Geometry: see drawing. Coordinates: mm, zero at the bounding-box minimum. A direction names the side the tool comes from. Give positions to 0.01 mm unless a question says otherwise; leave off trailing zeros. Write each loop counter-clockwise with the first axis right and the second up, starting at its lowest first coordinate (ties: lowest second). Pieces come first, ordered by that corner, then holes. Notation, with made-up numbers: (79, 89) -> (89, 89) arc R16 cw to (89, 99) -> close; hole circle Ø9 at (88.25, 84). An arc over 180 degrees is marked (long way). Use CSV: the item, a comma, the result in double quotes. Start each with the question number.
1) Section D-D (y = 21.5). Output: boundary loops of the cut face in (x, z), plus the area to 3 significant figures.
2) Set-up query: the marked faces 1, 2 and 3. Return all of +Z, -Z, +X, -X, +Y, -Y with unobstructed straight access to the full face (end or side cutting, diameter ignored); none if empty.
3) Section A-A (z = 21.5). Output: boundary loops of the cut face in (x, y).
4) Contact query for flat-ended pins moving along their axis: P1, Ø5, axis at x = 6, z = 19.5, coming from the +Y side; P2, Ø2, axis at x = 16, z = 18.5, coming from the -Y side; P3, Ø5, axis at x = 5, y = 29.5, coming from the +Z side. Output: stop coordinate, or through.
5) Section B-B (x = 31.5). Output: boundary loops of the cut face in (y, z), plus the area to 3 significant figures.
6) Material intervals for line 1 (Y direction, x = 8.5, z = 20); line 2 (Y direction, x = 47, z = 24.5), sorted ascending. Write a range as [from, to].
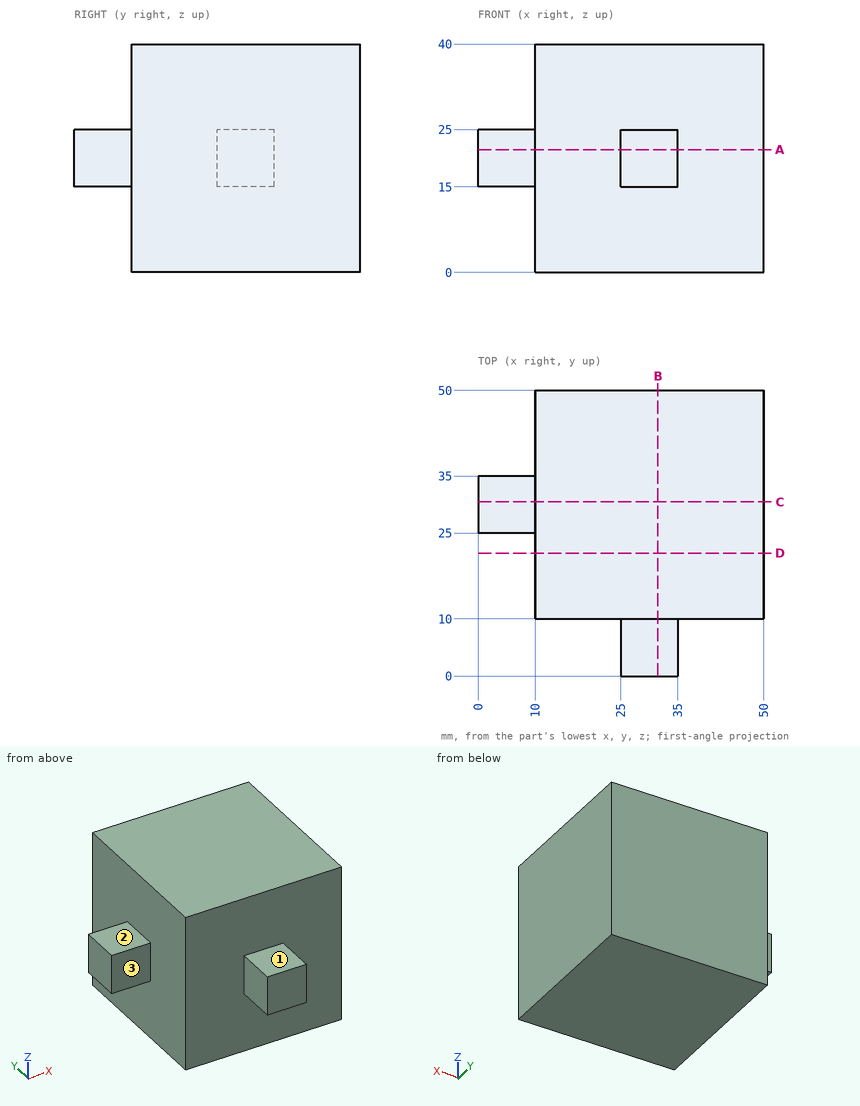
Answers follow:
1,outline,"(10, 0) -> (50, 0) -> (50, 40) -> (10, 40) -> close"
1,area,"1,600 mm^2"
2,face 1,"+Z, +X, -X, -Y"
2,face 2,"+Z, -X, +Y, -Y"
2,face 3,"+Z, -Z, -X, -Y"
3,outline,"(0, 25) -> (10, 25) -> (10, 10) -> (25, 10) -> (25, 0) -> (35, 0) -> (35, 10) -> (50, 10) -> (50, 50) -> (10, 50) -> (10, 35) -> (0, 35) -> close"
4,P1,"stops at y = 35"
4,P2,"stops at y = 10"
4,P3,"stops at z = 25"
5,outline,"(0, 15) -> (10, 15) -> (10, 0) -> (50, 0) -> (50, 40) -> (10, 40) -> (10, 25) -> (0, 25) -> close"
5,area,"1,700 mm^2"
6,line 1,"y = [25, 35]"
6,line 2,"y = [10, 50]"
